The listing builds one solid part. Answer for the finished solid, in the listing's coordinates (mm). A direction names the side the tool comes from. Coordinates: 2 decimals unless noted, no trailing zeros. Loops run counter-clockwise (first coordinate to the right, second up) from the corner with the lowest first, then second, coordinate; pieces in that order, holes last. Notation, with made-up numbers: (40.25, 41) - (67.25, 41) arc R16 cw to (67.25, 48) - close; hole circle Ø2 at (-22.5, 78). An arc over 180 degrees is marked (long way). Put each result on its own line as item: value.
Autodesk Inventor part; units mm, degrees
ref_plane "YZ Plane" through (0, 0, 0) normal (1, 0, 0) x (0, 1, 0)
ref_plane "XZ Plane" through (0, 0, 0) normal (0, 1, 0) x (-1, 0, 0)
ref_plane "XY Plane" through (0, 0, 0) normal (0, 0, 1) x (1, 0, 0)
sketch "Sketch1" plane through (0, 0, 0) normal (0, 0, 1) x (1, 0, 0)
  line L0 (-55, 4) -> (55, 4)
  line L1 (55, 4) -> (55, -4)
  line L2 (55, -4) -> (-55, -4)
  line L3 (-55, -4) -> (-55, 4)
  line L4 (-55, 4) -> (55, -4) construction
  line L5 (55, 4) -> (-55, -4) construction
  point P0 (0, 0)
  dimension "d0" = 110
  dimension "d1" = 8
extrude "Extrusion1" add sketch "Sketch1" along normal blind 37
sketch "Sketch2" plane through (0, 0, 37) normal (0, 0, 1) x (1, 0, 0)
  line L0 (-55, 4) -> (-55, -4)
  line L1 (55, -4) -> (55, 4)
  point P0 (0, 0)
  point P1 (-49, 0)
  point P2 (0, 0)
  point P3 (49, 0)
  dimension "d4" = 6
  dimension "d5" = 6
hole "Hole1" at (-49, 0, 37) at (0, 0, 37) at (49, 0, 37) direction (0, 0, -1) diameter 2.459 depth 8 tip angle 118
sketch "Sketch3" plane through (0, 0, 0) normal (0, 0, -1) x (-1, 0, 0)
  circle A0 centre (-49, 0) radius 1.2295
  circle A1 centre (0, 0) radius 1.2295
  circle A2 centre (49, 0) radius 1.2295
hole "Hole2" at (49, 0, 0) at (0, 0, 0) at (-49, 0, 0) direction (0, 0, 1) diameter 2.459 depth 8.8 tip angle 118
sketch "Sketch4" plane through (-55, -4, 0) normal (0, -1, 0) x (1, 0, 0)
  line L0 (18.55, 31.1) -> (31.45, 31.1)
  line L1 (31.45, 31.1) -> (31.45, 12)
  line L2 (31.45, 12) -> (18.55, 12)
  line L3 (18.55, 12) -> (18.55, 31.1)
  line L4 (18.55, 31.1) -> (31.45, 12) construction
  line L5 (31.45, 31.1) -> (18.55, 12) construction
  line L6 (110, 0) -> (0, 0)
  line L7 (0, 0) -> (0, 37)
  line L8 (110, 0) -> (110, 37)
  point P0 (55, 0)
  point P1 (25, 21.55)
  dimension "d21" = 12.9
  dimension "d22" = 19.1
  dimension "d23" = 12
  dimension "d29" = 85
extrude "Extrusion2" cut sketch "Sketch4" against normal blind 10
fillet "Fillet3" radius 0.75 4 edges at (-23.55, 0, 31.1) (-36.45, 0, 31.1) (-36.45, 0, 12) (-23.55, 0, 12)
sketch "Sketch5" plane through (-55, 4, 0) normal (0, 1, 0) x (1, 0, 0)
  line L0 (30.7, -31.1) -> (19.3, -31.1)
  line L1 (31.45, -12.75) -> (31.45, -30.35)
  line L2 (32.5, -32.05) -> (17.5, -32.05)
  line L3 (17.5, -32.05) -> (17.5, -11.05)
  line L4 (17.5, -11.05) -> (32.5, -11.05)
  line L5 (32.5, -11.05) -> (32.5, -32.05)
  line L6 (32.5, -32.05) -> (17.5, -11.05) construction
  line L7 (17.5, -32.05) -> (32.5, -11.05) construction
  point P0 (55, 0)
  point P1 (25, -21.55)
  dimension "d33" = 9.55
  dimension "d34" = 6.45
  dimension "d35" = 15
  dimension "d36" = 21
extrude "Extrusion3" cut sketch "Sketch5" against normal blind 5
sketch "Sketch6" plane through (-55, 4, 0) normal (0, 1, 0) x (1, 0, 0)
  line L0 (32.5, -32.05) -> (17.5, -32.05)
  line L1 (17.5, -32.05) -> (17.5, -11.05)
  line L2 (17.5, -11.05) -> (32.5, -11.05)
  point P0 (55, 0)
hole "Hole3" at (-22.5, 4, 32.05) at (-37.5, 4, 32.05) at (-37.5, 4, 11.05) at (-22.5, 4, 11.05) direction (0, -1, 0) diameter 1.5 depth 5
properties part number "side" material "Aluminum 6061"
1) Straight lines are drawn through the part: L1, parallel to Y at x = 0, z = 6.5; L2, parallel to X at y = 0, z = 7.5; L3, parallel to X at y = -1.25, z = 16. For each, find the intervals that lie inside material, in ascending order. Write a range as [from, to].
Found:
L1: y = [-4, -1.23], [1.23, 4]
L2: x = [-55, -50.23], [-47.77, -1.23], [1.23, 47.77], [50.23, 55]
L3: x = [-55, -36.45], [-23.55, 55]
2) The part is cut by section D-D (y = 2.5). Give the vertices of the cut face in (x, z).
Found:
outline: (-55, 0) - (55, 0) - (55, 37) - (-55, 37) - close; hole (-37.5, 11.8) arc R0.75 ccw (long way) to (-36.75, 11.05) - (-23.25, 11.05) arc R0.75 ccw (long way) to (-22.5, 11.8) - (-22.5, 31.3) arc R0.75 ccw (long way) to (-23.25, 32.05) - (-36.75, 32.05) arc R0.75 ccw (long way) to (-37.5, 31.3) - close
3) For faces 1 (the face through (0.748, -0.976, 4.462)), 2 (the face through (-50.22, 0.16, 32.94)), 3 (the face through (-23.55, -3, 22)), 4 (the face through (-37.5, 2, 22)), determine the directions among +Z, -Z, +X, -X, +Y, -Y from which every point of the face is accessible in a straight line to the end or side of a thin tool.
Found:
face 1: -Z
face 2: +Z
face 3: +Y, -Y
face 4: +Y
4) Each of these flat-tipped pins is pushed along its axis until it touches: pin 1 (2 mm diameter, centred on x = 49, y = 0, fed in from -Z); pin 2 (2 mm diameter, centred on x = 49, y = 0, fed in from +Z); pin 3 (0.9 mm diameter, centred on x = -37.5, z = 11.05, fed in from +Y). Where does it stop, or does it pass through?
Found:
pin 1: stops at z = 8.94
pin 2: stops at z = 28.86
pin 3: stops at y = -1
5) For a pull along Z with two mould halves and no side action, classify faces 5 (the face through (48.81, -0.1, 28.39)), 6 (the face through (-30, 2, 32.05)), 7 (the face through (47.78, -0.16, 4.46)) as pulls with the +Z half, pulls with the -Z half, needs draft (parallel to the pull), parting line crosses it, or undercut.
Found:
face 5: pulls with the +Z half
face 6: undercut
face 7: needs draft
6) The part is cut by section C-C (y = -2.25). Give the vertices of the cut face in (x, z), and give its area (3 significant figures).
Found:
outline: (-55, 0) - (55, 0) - (55, 37) - (-55, 37) - close; hole (-36.45, 12.75) arc R0.75 ccw to (-35.7, 12) - (-24.3, 12) arc R0.75 ccw to (-23.55, 12.75) - (-23.55, 30.35) arc R0.75 ccw to (-24.3, 31.1) - (-35.7, 31.1) arc R0.75 ccw to (-36.45, 30.35) - close
area: 3,820 mm^2
7) The part is cut by section B-B (z = 6). Give the vertices of the cut face in (x, y), and give its area (3 significant figures).
Found:
outline: (-55, -4) - (55, -4) - (55, 4) - (-55, 4) - close; hole circle Ø2.46 at (-49, 0); hole circle Ø2.46 at (0, 0); hole circle Ø2.46 at (49, 0)
area: 866 mm^2
8) The part is cut by section A-A (x = -29.5). Give the vertices of the cut face in (y, z), and give its area (3 significant figures).
Found:
outline: (-4, 0) - (4, 0) - (4, 11.05) - (-1, 11.05) - (-1, 12) - (-4, 12) - close; (-4, 31.1) - (-1, 31.1) - (-1, 32.05) - (4, 32.05) - (4, 37) - (-4, 37) - close
area: 134 mm^2
